Autodesk Inventor part; units mm, degrees
ref_plane "YZ Plane" through (0, 0, 0) normal (1, 0, 0) x (0, 1, 0)
ref_plane "XZ Plane" through (0, 0, 0) normal (0, 1, 0) x (-1, 0, 0)
ref_plane "XY Plane" through (0, 0, 0) normal (0, 0, 1) x (1, 0, 0)
sketch "Sketch1" plane through (0, 0, 0) normal (0, 0, 1) x (1, 0, 0)
  line L0 (0, 114) -> (0, -114) construction
  line L1 (-9.4, 0) -> (9.4, 0)
  line L2 (-5, 7.5) -> (5, 7.5)
  arc A0 (-9.4, 0) -> (-5, 7.5) centre (-24.038, 13.6283) ccw
  arc A1 (5, 7.5) -> (9.4, 0) centre (24.038, 13.6283) ccw
  point P0 (0, 0)
  point P1 (0, 0)
  point P2 (0, 7.5)
  dimension "d9" = 18.8
  dimension "d10" = 10
  dimension "d11" = 7.5
  dimension "d13" = 20
extrude "Extrusion1" add sketch "Sketch1" along normal blind 4.6
sketch "Sketch2" plane through (-9.4, 0, 0) normal (0, -1, 0) x (1, 0, 0)
  line L0 (-8.6, 6.8) -> (27.4, 6.8)
  line L1 (27.4, 6.8) -> (27.4, -2.2)
  line L2 (27.4, -2.2) -> (-8.6, -2.2)
  line L3 (-8.6, -2.2) -> (-8.6, 6.8)
  line L4 (0, 4.6) -> (18.8, 4.6)
  line L5 (0, 0) -> (18.8, 0)
  line L6 (0, 0) -> (0, 4.6)
  line L7 (18.8, 0) -> (18.8, 4.6)
  point P0 (9.4, 0)
  point P1 (0, 2.3)
  dimension "d16" = 36
  dimension "d17" = 9
  dimension "d18" = 2.2
  dimension "d19" = 2.2
  dimension "d20" = 8.6
  dimension "d21" = 8.6
extrude "Extrusion2" add sketch "Sketch2" along normal blind 4.5 contours L0 L1 L2 L3 | L4 L7 L5 L6
fillet "Fillet1" radius 2 4 edges at (0, 0, 4.6) (9.4, 0, 2.3) (0, 0, 0) (-9.4, 0, 2.3)
sketch "Sketch3" plane through (-5, 7.5, 0) normal (0, 1, 0) x (1, 0, 0)
  circle A0 centre (5, -2.3) radius 2
  circle A1 centre (5, -2.3) radius 1.75
  line L0 (10, -4.6) -> (0, -4.6)
  line L1 (10, 0) -> (0, 0)
  line L2 (0, 0) -> (0, -4.6)
  point P0 (5, 0)
  dimension "d25" = 4
  dimension "d26" = 3.5
  dimension "d27" = 2.3
  dimension "d28" = 2.3
  dimension "d29" = 5
extrude "Extrusion3" add sketch "Sketch3" along normal blind 21
sketch "Sketch4" plane through (-9.4, 0, 0) normal (0, 1, 0) x (1, 0, 0)
  circle A0 centre (-4.1, -2.3) radius 2
  circle A1 centre (22.9, -2.3) radius 2
  line L0 (-8.6, 2.2) -> (27.4, 2.2)
  circle A2 centre (9.4, -2.3) radius 1.75
  circle A3 centre (9.4, -2.3) radius 2
  circle A4 centre (9.4, -2.3) radius 1.75
  circle A5 centre (9.4, -2.3) radius 1.75
  point P0 (9.4, 0)
  dimension "d32" = 4
  dimension "d33" = 4
  dimension "d34" = 4.5
  dimension "d35" = 4.5
  dimension "d36" = 3.5
  dimension "d37" = 13.5
  dimension "d38" = 13.5
hole "Hole1" at (-13.5, 0, 2.3) at (13.5, 0, 2.3) direction (0, -1, 0) diameter 4 end through all
equation "\"d38\" = d37"
properties part number "HUDSON-1-12 LEAFSPING SOLID EQUALISER"
CAD build for the part. Positions are in the model's coordinates, mm. A direction names the side the tool comes from. Round coordinates to 2 decimals unless told otherwise and drop trailing zeros. Loops run counter-clockwise (first coordinate to the right, second up) from the corner with the lowest first, then second, coordinate; pieces in that order, holes last. Notation, with made-up numbers: M -24.75,75 L 6.25,75 A22 ccw 6.25,84 Z; hole C 20.25,80 d8. An arc over 180 degrees is marked long. Return JSON: item names as keys, results as strings. Group by question number.
(1) Saw through at A-A, the plane x = 13.5. List the corners of the cut face in (y, z), and give its area (3 significant figures).
(2) Saw through at B-B, the plane z = 1.5. List the corners of the cut face in (x, y).
(3) Saw through at C-C, the plane x = 0. List the corners of the cut face in (y, z), and give its area (3 significant figures).
(4) Mould opens along X. For faces 4 (the flat face through (0, 7.5, 2)), 5 (the cylindrical face through (-6.526, 3.967, 2.261)), 6 (the cylindrical face through (0.14, 0.6, -0.57)) say: +X half, -X half, draft (parallel to the pull), parting line (faces both ways), or undercut.
(5) Saw through at D-D, the plane y = 15. List the corners of the cut face in (x, z), and give its area (3 significant figures).
(6) Drop flat-ended pins along their axis: P1, Ø5, axis at y = 19.5, z = 0.5, coming from the +X side; P2, Ø1, axis at x = -1, z = 6, coming from the +Y side; P3, Ø3, axis at x = 1, y = 4, coming from the -Z side. Give the stop position or say it passes through.
(7) Wall check: probe 1 along X at (y, z) = (-1.4, 2.3); probe 2 along Z at (x, y) = (0, 21); probe 3 along X at (y, z) = (12, 2.3). Give the ranges that are in metal, low to high. Write a range as [from, to].
(8) Tool access for faces 1 (the flat face through (0, -4.5, 2)), 2 (the cylindrical face through (-0.26, 17.853, 4.283)), 3 (the flat face through (0, 5, 4.6)): list every direction of +Z, -Z, +X, -X, +Y, -Y with a clear straight run to the whole face (end or side of a thin tool).
Answer list:
{
 "1": {"outline": "M -4.5,-2.2 L 0,-2.2 L 0,0.3 L -4.5,0.3 Z; M -4.5,4.3 L 0,4.3 L 0,6.8 L -4.5,6.8 Z", "area": "22.5 mm2"},
 "2": {"outline": "M -18,-4.5 L -15.33,-4.5 L -15.33,0 L -18,0 Z; M -11.67,-4.5 L 11.67,-4.5 L 11.67,0 L 10.3,0 A2 cw 8.77,0.71 A20 cw 5,7.5 L 1.83,7.5 L 1.83,28.5 L 1.56,28.5 L 1.56,7.5 L -1.56,7.5 L -1.56,28.5 L -1.83,28.5 L -1.83,7.5 L -5,7.5 A20 cw -8.77,0.71 A2 cw -10.3,0 L -11.67,0 Z; M 15.33,-4.5 L 18,-4.5 L 18,0 L 15.33,0 Z"},
 "3": {"outline": "M -4.5,-2.2 L 0,-2.2 L 0,-2 A2 cw 2,0 L 7.5,0 L 7.5,0.3 L 28.5,0.3 L 28.5,0.55 L 7.5,0.55 L 7.5,4.05 L 28.5,4.05 L 28.5,4.3 L 7.5,4.3 L 7.5,4.6 L 2,4.6 A2 cw 0,6.6 L 0,6.8 L -4.5,6.8 Z", "area": "87.2 mm2"},
 "4": {"face 4": "undercut", "face 5": "-X half", "face 6": "draft"},
 "5": {"outline": "C 0,2.3 d4; hole C 0,2.3 d3.5", "area": "2.95 mm2"},
 "6": {"P1": "x = 2", "P2": "y = 0.33", "P3": "z = 0"},
 "7": {"probe 1": "[-18, -15.5], [-11.5, 11.5], [15.5, 18]", "probe 2": "[0.3, 0.55], [4.05, 4.3]", "probe 3": "[-2, -1.75], [1.75, 2]"},
 "8": {"face 1": "+Z, -Z, +X, -X, -Y", "face 2": "+Y", "face 3": "+Z, +X, -X, +Y"}
}
